from build123d import *

# Parameters (mm, degrees)
SKETCH_1_W          = 156.75
SKETCH_1_H          = 105.271994628
EXTRUDE_1_DEPTH     = 12.2
SKETCH_2_W          = 7.639581741
SKETCH_2_H          = 13.89014237
CUT_EXTRUDE_1_DEPTH = 6.1
SKETCH_4_R          = 5.5
EXTRUDE_2_DEPTH     = 18
EXTRUDE_2_TAPER     = 5
CUT_EXTRUDE_2_REACH = 20
SKETCH_6_R          = 1.55
SKETCH_7_W          = 7
SKETCH_7_H          = 3.5
CUT_EXTRUDE_3_DEPTH = 9.1
SKETCH_8_W          = 140.75
SKETCH_8_H          = 89.271994628
CUT_EXTRUDE_4_DEPTH = 13.2


with BuildPart() as part:
    # ｽｹｯﾁ1 → ﾎﾞｽ - 押し出し1 (new body)
    with BuildSketch(Plane(origin=(0, 0, 0), x_dir=(1, 0, 0), z_dir=(0, 1, 0))):
        Rectangle(SKETCH_1_W, SKETCH_1_H)
    extrude(amount=EXTRUDE_1_DEPTH)

    # ｽｹｯﾁ2 → ｶｯﾄ - 押し出し1 (cut)
    with BuildSketch(Plane(origin=(0, 12.2, 0), x_dir=(1, 0, 0), z_dir=(0, 1, 0))):
        with BuildLine():
            ThreePointArc((-44.016, 13.890145056), (-40.196209129, 16.500447871), (-36.376418259, 13.890145056))
            Line((-36.376418259, 13.890145056), (-44.016, 13.890145056))
        make_face()
        with Locations((-40.19620913, 6.945073871)):
            Rectangle(SKETCH_2_W, SKETCH_2_H)
        with BuildLine():
            Line((-44.016, 2.686e-06), (-36.376418259, 2.686e-06))
            ThreePointArc((-36.376418259, 2.686e-06), (-40.196209129, -2.610300128), (-44.016, 2.686e-06))
        make_face()
        with BuildLine():
            Line((44.016, 13.890145056), (36.376418259, 13.890145056))
            ThreePointArc((36.376418259, 13.890145056), (40.196209129, 16.500447871), (44.016, 13.890145056))
        make_face()
        with Locations((40.19620913, 6.945073871)):
            Rectangle(SKETCH_2_W, SKETCH_2_H)
        with BuildLine():
            ThreePointArc((44.016, 2.686e-06), (40.196209129, -2.610300128), (36.376418259, 2.686e-06))
            Line((36.376418259, 2.686e-06), (44.016, 2.686e-06))
        make_face()
    extrude(amount=-CUT_EXTRUDE_1_DEPTH, mode=Mode.SUBTRACT)

    # ｽｹｯﾁ4 → ﾎﾞｽ - 押し出し2 (add)
    with BuildSketch(Plane.XY.offset(52.635997314)):
        with Locations((-22.875, 6.1)):
            Circle(SKETCH_4_R)
        with Locations((22.875, 6.1)):
            Circle(SKETCH_4_R)
    extrude(amount=EXTRUDE_2_DEPTH, taper=EXTRUDE_2_TAPER)

    # ｽｹｯﾁ6 → ｶｯﾄ - 押し出し2 (cut, up to next)
    with BuildSketch(Plane.XY.offset(52.635997314), mode=Mode.PRIVATE) as cut_extrude_2_sk1:
        with Locations((-22.875, 6.1)):
            Circle(SKETCH_6_R)
    cut_extrude_2_tool1 = extrude(cut_extrude_2_sk1.sketch, amount=CUT_EXTRUDE_2_REACH, mode=Mode.PRIVATE) & part.part
    add(cut_extrude_2_tool1.solids().sort_by_distance((-22.875, 6.1, 52.635997))[0], mode=Mode.SUBTRACT)
    # ｽｹｯﾁ6 → ｶｯﾄ - 押し出し2 (cut, up to next)
    with BuildSketch(Plane.XY.offset(52.635997314), mode=Mode.PRIVATE) as cut_extrude_2_sk2:
        with Locations((22.875, 6.1)):
            Circle(SKETCH_6_R)
    cut_extrude_2_tool2 = extrude(cut_extrude_2_sk2.sketch, amount=CUT_EXTRUDE_2_REACH, mode=Mode.PRIVATE) & part.part
    add(cut_extrude_2_tool2.solids().sort_by_distance((22.875, 6.1, 52.635997))[0], mode=Mode.SUBTRACT)

    # ｽｹｯﾁ7 → ｶｯﾄ - 押し出し3 (cut)
    with BuildSketch(Plane(origin=(0, 0, 0), x_dir=(1, 0, 0), z_dir=(0, 1, 0))):
        with Locations((-22.875, -58.885997314)):
            Rectangle(SKETCH_7_W, SKETCH_7_H)
        with Locations((22.875, -58.885997314)):
            Rectangle(SKETCH_7_W, SKETCH_7_H)
    extrude(amount=CUT_EXTRUDE_3_DEPTH, mode=Mode.SUBTRACT)

    # ｽｹｯﾁ8 → ｶｯﾄ - 押し出し4 (cut, through all)
    with BuildSketch(Plane(origin=(0, 0, 0), x_dir=(-1, 0, 0), z_dir=(0, -1, 0))):
        Rectangle(SKETCH_8_W, SKETCH_8_H)
    extrude(amount=-CUT_EXTRUDE_4_DEPTH, mode=Mode.SUBTRACT)


solid = part.part
Verification items for the finished model (mm, model axes). A direction names the side the tool comes from. Round coordinates to 2 decimals unless told otherwise and drop trailing zeros. Loops run counter-clockwise (first coordinate to the right, second up) from the corner with the lowest first, then second, coordinate; pieces in that order, holes last. Notation, with made-up numbers: M 23,9.25 L 55,9.25 A30 ccw 55,44.25 Z; hole C -17,74 d1. An arc over 180 degrees is marked long. Write each question's results on one line, items separated by ' | '.
1) Gauge pin test, flat ends, axial feed: P1, Ø5, axis at x = 22.875, y = 6.1, coming from the +Z side; P2, Ø5, axis at x = -6.5, y = 3, coming from the +Z side; P3, Ø1, axis at x = 24.5, z = 59.5, coming from the -Y side; P4, Ø3, axis at y = 5.5, z = 59, coming from the -X side. Record the tip position at first contact, or that the pin passes through.
Checks:
P1: stops at z = 70.64 | P2: stops at z = 52.64 | P3: stops at y = 9.1 | P4: stops at x = -27.94
2) Mould release check, pull along Z, two halves, no side actions. Record for faces 4 (the conical face through (-23.49, 10.76, 61.76)), 5 (the flat face through (-19.375, 6, 59)), 6 (the cylindrical face through (24.31, 5.51, 65.57)): released by +Z, released by -Z, zero draft, split by the parting line, or undercut.
Checks:
face 4: released by +Z | face 5: undercut | face 6: zero draft
3) Section check A-A on z = -17.5. Record the boundary of the cut face in (x, y) (3 decimals), then the cut area to 3 significant figures.
Checks:
outline: M -78.375,0 L -70.375,0 L -70.375,12.2 L -78.375,12.2 Z; M 70.375,0 L 78.375,0 L 78.375,12.2 L 70.375,12.2 Z | area: 195 mm2
4) Access from +Z, -Z, +X, -X, +Y, -Y to the whole of each face (thin tool, end or side, straight path). Record for faces 1 (the cylindrical face through (-21.44, 5.51, 54.85)), 2 (the flat face through (23, 9.1, 59)), 3 (the flat face through (1, 6, -44.636)).
Checks:
face 1: +Z | face 2: -Y | face 3: +Y, -Y
5) Scan lines: L1, parallel to Z at x = 1, y = 7.5; L2, parallel to X at y = 5, z = -32 (3 decimals); L3, parallel to Z at x = -24, y = 4.5. Record each from-to range of solid material in increasing order. Write a range as from..to.
Checks:
L1: z = -52.64..-44.64, 44.64..52.64 | L2: x = -78.375..-70.375, 70.375..78.375 | L3: z = -52.64..-44.64, 44.64..57.14, 60.64..70.64
6) Section check B-B on x = 14. Record the boundary of the cut face in (y, z), then the cut area to 3 significant figures.
Checks:
outline: M 0,-52.64 L 12.2,-52.64 L 12.2,-44.64 L 0,-44.64 Z; M 0,44.64 L 12.2,44.64 L 12.2,52.64 L 0,52.64 Z | area: 195 mm2
